from build123d import *

# Parameters (mm, degrees)
SKETCH1_W           = 24
SKETCH1_H           = 13
BOSS_EXTRUDE1_DEPTH = 10
CUT_EXTRUDE2_DEPTH  = 11
FILLET1_R           = 10


with BuildPart() as part:
    # Sketch1 → Boss-Extrude1 (new body)
    with BuildSketch(Plane.XY):
        with Locations((12, 6.5)):
            Rectangle(SKETCH1_W, SKETCH1_H)
        Polygon((24, 13), (34.5, 13), (34.5, 20), (-10.5, 20), (-10.5, 13), (0, 13), align=None)
    extrude(amount=BOSS_EXTRUDE1_DEPTH)

    # Sketch2 → Cut-Extrude2 (cut, through all)
    with BuildSketch(Plane(origin=(0, 0, 0), x_dir=(-1, 0, 0), z_dir=(0, 0, -1))):
        with BuildLine():
            Line((0, 20), (-24, 20))
            ThreePointArc((-24, 20), (-12, 12), (0, 20))
        make_face()
    extrude(amount=-CUT_EXTRUDE2_DEPTH, mode=Mode.SUBTRACT)

    # Fillet1
    fillet1_edges = [part.edges().sort_by_distance(p)[0] for p in [
        (0, 20, 5),
        (24, 20, 5),
    ]]
    fillet(fillet1_edges, radius=FILLET1_R)


solid = part.part
Build history of the part. All positions in model axes, mm. A direction names the side the tool comes from. Give positions to 0.01 mm unless a question says otherwise; leave off trailing zeros. Order: outer loops, then holes, each group sorted by start corner. A loop starts at its lowest first (then second) coordinate and runs counter-clockwise, first axis right, second up. Notation, with made-up numbers: M -8,89 L 8,89 A30 cw 8,111 Z; hole C 57,50.25 d6. An arc over 180 degrees is marked long. Put each result on its own line as item: value.
Item 1: Cut at B-B on z = 5.25. Write the cut outline in (x, y), then the cut area to 3 significant figures.
Results are:
outline: M -10.5,13 L 0,13 L 0,0 L 24,0 L 24,13 L 34.5,13 L 34.5,20 L 29.44,20 A10 ccw 21.85,16.52 A13 cw 2.15,16.52 A10 ccw -5.44,20 L -10.5,20 Z
area: 480 mm2
Item 2: Cut at C-C on y = 16. Write the cut outline in (x, z).
Results are:
outline: M -10.5,0 L 2.62,0 L 2.62,10 L -10.5,10 Z; M 21.38,0 L 34.5,0 L 34.5,10 L 21.38,10 Z
Item 3: Which spindle directions (+Z, -Z, +X, -X, +Y, -Y) get a long thin tool onto all of the face, cutting with end or side? Do faces 1 (the face through (-1.32, 19.114, 5.07)), 2 (the face through (24, 6, 5)), 3 (the face through (-5, 13, 5)), 4 (the face through (12, 10, 10)). Say none if no direction does.
Results are:
face 1: +Z, -Z, +Y
face 2: +Z, -Z, +X, -Y
face 3: +Z, -Z, -X, -Y
face 4: +Z, +X, -X, +Y, -Y
Item 4: Wall check: probe 1 along X at (y, z) = (6.75, 4.5); probe 2 along X at (y, z) = (16.25, 2.5); probe 3 along Y at (x, z) = (32.5, 2.25). Give the ranges that are in metal, low to high.
Results are:
probe 1: 0 to 24
probe 2: -10.5 to 2.39, 21.61 to 34.5
probe 3: 13 to 20
Item 5: Cut at D-D on x = -7.5. Write the cut outline in (y, z).
Results are:
outline: M 13,0 L 20,0 L 20,10 L 13,10 Z
Item 6: Drop a flat-ended pin along its axis: pin 1 Ø3 at (y, z) = (8.5, 3) entering from +X. Give the stop position or say it passes through.
Results are:
pin 1: x = 24
Item 7: Pull direction X, two halves, no side cores. Call faces 5 (the face through (12, 0, 5)), 6 (the face through (0, 6, 5)), 7 (the face through (25.211, 19.064, 5.07)): +X half, -X half, draft (parallel to the pull), parting line (faces both ways), or undercut.
Results are:
face 5: draft
face 6: -X half
face 7: undercut
Item 8: Cut at A-A on y = 13.75. Write the cut outline in (x, z), then the cut area to 3 significant figures.
Results are:
outline: M -10.5,0 L 5.49,0 L 5.49,10 L -10.5,10 Z; M 18.51,0 L 34.5,0 L 34.5,10 L 18.51,10 Z
area: 320 mm2
